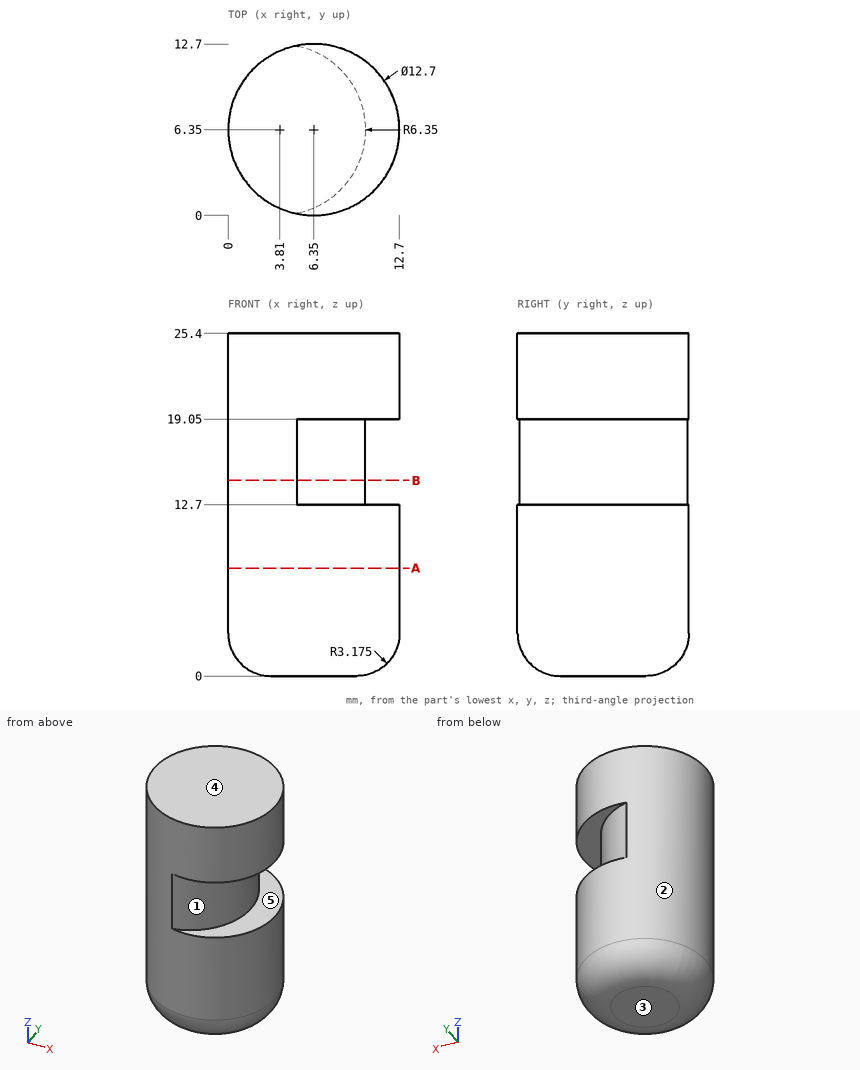
Answer from the drawing. Dimensions are ordinates in mm from the lowest x, y and z of the part. A direction names the side the tool comes from. Coordinates: 2 decimals unless noted, no trailing zeros. Order: outer loops, then holes, each group sorted by start corner. A loop starts at its lowest first (then second) coordinate and runs counter-clockwise, first axis right, second up. Notation, with made-up numbers: (65, -15) -> (73, -15) arc R21 ccw to (73, 7) -> close; hole circle Ø5 at (30.5, -10.5). An arc over 180 degrees is marked (long way). Answer as a JSON object with one key per item and string values.
1) Each of these flat-tipped pins is pushed along its axis until it touches: pin 1 (1 mm diameter, centred on x = 10, y = 3, fed in from -Z); pin 2 (1 mm diameter, centred on y = 8.5, z = 18, fed in from -X); pin 3 (5 mm diameter, centred on y = 2.5, z = 3.5, fed in from -X). Where does it stop, or does it pass through?
Model answer:
{"pin 1": "stops at z = 0.27", "pin 2": "stops at x = 0.22", "pin 3": "stops at x = 0.15"}
2) The mould has two halves that part along Z. Classify the marked faces 3, 4 and 5: released by +Z, released by -Z, zero draft, split by the parting line, or undercut.
Model answer:
{"face 3": "released by -Z", "face 4": "released by +Z", "face 5": "undercut"}
3) A cutting plane is placed at B-B, the plane z = 14.5. Determine the outline of the cut face in (x, y), plus the area to 3 significant figures.
Model answer:
{"outline": "(5.08, 0.13) arc R6.35 ccw to (5.08, 12.57) arc R6.35 ccw to start", "area": "94.6 mm²"}
4) A cutting plane is placed at A-A, the plane z = 8. Determine the outline of the cut face in (x, y).
Model answer:
{"outline": "circle Ø12.7 at (6.35, 6.35)"}
5) A tool of negligible diameter and unlimited length cuts with its end or side. For the marked faces 1 and 2, from which of +Z, -Z, +X, -X, +Y, -Y can it reach the whole face along a straight path? Write none if from no direction.
Model answer:
{"face 1": "+X", "face 2": "+Z, -Z"}
6) Consider line 1 along Z through (x, y) = (11.5, 3.25); line 2 along Z through (x, y) = (9.25, 2.5); line 3 along Y through (x, z) = (6.25, 22.75). Determine where each line is inside the solid, lowest interval first. Write a range as from..to.
Model answer:
{"line 1": "z = 1.75..12.7, 19.05..25.4", "line 2": "z = 0.46..12.7, 19.05..25.4", "line 3": "y = 0..12.7"}
